from build123d import *

# Parameters (mm, degrees)
F0_R     = 6.35
F0_R_2   = 15.875
F1_DEPTH = 6.35


with BuildPart() as f1:
    # F0 (on Front) → F1 (new body)
    with BuildSketch(Plane.XZ):
        Polygon((50.8, -31.75), (50.8, 12.7), (14.804928, 31.75), (-16.945072, 31.75), (-50.8, 12.7), (-50.8, -31.75), align=None)
        with Locations((-31.75, -12.7)):
            Circle(F0_R, mode=Mode.SUBTRACT)
        with Locations((31.75, -12.7)):
            Circle(F0_R, mode=Mode.SUBTRACT)
        Circle(F0_R_2, mode=Mode.SUBTRACT)
    extrude(amount=F1_DEPTH)


solid = f1.part
The model under review builds one solid part; all positions refer to its coordinate system, in mm. Give positions to 0.01 mm unless a question says otherwise; leave off trailing zeros. Loops run counter-clockwise (first coordinate to the right, second up) from the corner with the lowest first, then second, coordinate; pieces in that order, holes last. Notation, with made-up numbers: (-21, 23) -> (-7, 23) arc R15 ccw to (-7, 31) -> close; hole circle Ø10 at (-3.75, 6). An arc over 180 degrees is marked (long way). Answer as a JSON object with one key per item and string values. Group by question number.
Q1. Wall thickness on line 1 along X through (y, z) = (-0.5, -17.5); line 2 along Z through (x, y) = (0, -1.5) (3 decimals); line 3 along X through (y, z) = (-0.5, -11): over which ranges is each line inside the solid? List them lowest first.
Q2. Take a section at A-A (z = 0). Write out the cut boundary in (x, y) (3 decimals), plus the area to 3 significant figures.
Q3. Insertion check: pin 1 (1 mm diameter, centred on x = -29.5, z = -18.5, fed in from -Y); pin 2 (2 mm diameter, centred on x = 22, y = -4, fed in from +Z). Each pin has a flat end and moves straight along its axis. Give the tip position at first contact, or say it passes through.
Q4. Take a section at C-C (y = -3). Write out the cut boundary in (x, z) (3 decimals), plus the area to 3 significant figures.
Q5. Take a section at B-B (x = 0). Write out the cut boundary in (y, z) (3 decimals), plus the area to 3 significant figures.
Q6. Take a section at D-D (x = 22.5). Write out the cut boundary in (y, z).
Q7. Draft analysis for pull direction Z (two halves, no side actions). For faces 1 (the flat face through (33.054, -3.131, 22.092)), 2 (the flat face through (-1, -3, -31.75)), 3 (the cylindrical face through (-25.884, -3.131, -15.132)), state which applies: pulls with the +Z half, pulls with the -Z half, needs draft (parallel to the pull), parting line crosses it, or undercut.
Answer below:
{
 "1": {"line 1": "x = -50.8 to -35.91, -27.59 to 27.59, 35.91 to 50.8", "line 2": "z = -31.75 to -15.875, 15.875 to 31.75", "line 3": "x = -50.8 to -37.87, -25.63 to -11.45, 11.45 to 25.63, 37.87 to 50.8"},
 "2": {"outline": "(-50.8, -6.35) -> (-15.875, -6.35) -> (-15.875, 0) -> (-50.8, 0) -> close; (15.875, -6.35) -> (50.8, -6.35) -> (50.8, 0) -> (15.875, 0) -> close", "area": "444 mm2"},
 "3": {"pin 1": "stops at y = -6.35", "pin 2": "stops at z = 28.47"},
 "4": {"outline": "(-50.8, -31.75) -> (50.8, -31.75) -> (50.8, 12.7) -> (14.805, 31.75) -> (-16.945, 31.75) -> (-50.8, 12.7) -> close; hole circle Ø12.7 at (-31.75, -12.7); hole circle Ø31.75 at (0, 0); hole circle Ø12.7 at (31.75, -12.7)", "area": "4,740 mm2"},
 "5": {"outline": "(-6.35, -31.75) -> (0, -31.75) -> (0, -15.875) -> (-6.35, -15.875) -> close; (-6.35, 15.875) -> (0, 15.875) -> (0, 31.75) -> (-6.35, 31.75) -> close", "area": "202 mm2"},
 "6": {"outline": "(-6.35, -31.75) -> (0, -31.75) -> (0, 27.68) -> (-6.35, 27.68) -> close"},
 "7": {"face 1": "pulls with the +Z half", "face 2": "pulls with the -Z half", "face 3": "undercut"}
}
